The listing builds one solid part. Answer for the finished solid, in the listing's coordinates (mm). Round coordinates to 2 decimals unless told otherwise and drop trailing zeros. Order: outer loops, then holes, each group sorted by start corner. A loop starts at its lowest first (then second) coordinate and runs counter-clockwise, first axis right, second up. Notation, with made-up numbers: (-20, 67.25) - (-4, 67.25) arc R10 ccw to (-4, 73.25) - close; hole circle Ø2 at (54.5, 70.5). An arc over 180 degrees is marked (long way). Write item = value, one per line.
from build123d import *

# Parameters (mm, degrees)
SKETCH1_W           = 20
SKETCH1_H           = 20
SKETCH1_R           = 5
BOSS_EXTRUDE1_DEPTH = 120
SKETCH2_R           = 7.5
BOSS_EXTRUDE2_DEPTH = 120


with BuildPart() as part:
    # Sketch1 → Boss-Extrude1 (new body)
    with BuildSketch(Plane.XY):
        Rectangle(SKETCH1_W, SKETCH1_H)
        Circle(SKETCH1_R, mode=Mode.SUBTRACT)
    extrude(amount=BOSS_EXTRUDE1_DEPTH)

    # Sketch2 → Boss-Extrude2 (add)
    with BuildSketch(Plane(origin=(0, 10, 0), x_dir=(1, 0, 0), z_dir=(0, 1, 0))):
        with Locations(Location((0, -60, 0), (0, 0, 90))):
            Circle(SKETCH2_R)
    extrude(amount=BOSS_EXTRUDE2_DEPTH)


solid = part.part
Q1. Section C-C on z = 49.5 is taken. Determine the outline of the cut face in (x, y), then the cut area to 3 significant figures.
Model answer:
outline = (-10, -10) - (10, -10) - (10, 10) - (-10, 10) - close; hole circle Ø10 at (0, 0)
area = 321 mm^2
Q2. Section B-B on y = 0 is taken. Determine the outline of the cut face in (x, z), then the cut area to 3 significant figures.
Model answer:
outline = (-10, 0) - (-5, 0) - (-5, 120) - (-10, 120) - close; (5, 0) - (10, 0) - (10, 120) - (5, 120) - close
area = 1,200 mm^2
Q3. Section A-A on x = 0 is taken. Determine the outline of the cut face in (y, z).
Model answer:
outline = (-10, 0) - (-5, 0) - (-5, 120) - (-10, 120) - close; (5, 0) - (10, 0) - (10, 52.5) - (130, 52.5) - (130, 67.5) - (10, 67.5) - (10, 120) - (5, 120) - close
Q4. Find the intervals of material crossed by line 1 (Y direction, x = 0, z = 46.5); line 2 (Y direction, x = 6.25, z = 112.5); line 3 (Y direction, x = -1.25, z = 86.5), in increasing order. Write a range as from..to.
Model answer:
line_1 = -10..-5, 5..10
line_2 = -10..10
line_3 = -10..-4.84, 4.84..10
Q5. Determine the mould class of faces 1 (the face through (-1.08, -4.88, 59.16)), 2 (the face through (-5.1, 69.2, 65.5)), 3 (the face through (10, 0, 59)) for opening direction X: released by +X, released by -X, zero draft, split by the parting line, or undercut.
Model answer:
face_1 = undercut
face_2 = split by the parting line
face_3 = released by +X
Q6. Section D-D on y = 19.5 is taken. Determine the outline of the cut face in (x, z).
Model answer:
outline = circle Ø15 at (0, 60)
Q7. Flat-ended cylindrical pins translate along their axes: P1, Ø12, axis at x = 7.5, z = 30, coming from the +Y side; P2, Ø12, axis at x = -7.5, y = 35.5, coming from the -Z side; P3, Ø8, axis at x = 7.5, y = 15.5, coming from the -Z side. Find the tip coordinate at first contact, or state that the pin passes through.
Model answer:
P1 = 10
P2 = 52.65
P3 = 53.37
